CAD build for the part. Positions are in the model's coordinates, mm. A direction names the side the tool comes from. Coordinates: 2 decimals unless noted, no trailing zeros. Write each loop counter-clockwise with the first axis right and the second up, starting at its lowest first coordinate (ties: lowest second). Pieces come first, ordered by that corner, then holes. Notation, with made-up numbers: M 46.5,-9 L 90.5,-9 A14 ccw 90.5,-5 Z; hole C -20,-36 d1. An arc over 180 degrees is marked long. Answer as CSV lines item,"result". Start each with the question number.
```python
from build123d import *

# Parameters (mm, degrees)
BOSS_EXTRU_1_DEPTH      = 132
ESQUISSE3_W             = 4.94012132
ESQUISSE3_H             = 40
ENL_V_MAT_EXTRU_2_DEPTH = 9
ESQUISSE4_R             = 1.3
ENL_V_MAT_EXTRU_3_DEPTH = 18
ESQUISSE5_W             = 6
ESQUISSE5_H             = 24
ENL_V_MAT_EXTRU_4_DEPTH = 8
BOSS_EXTRU_2_REACH      = 38.8
ESQUISSE7_W             = 2
ESQUISSE7_H             = 18
ENL_V_MAT_EXTRU_5_DEPTH = 15
ENL_V_MAT_EXTRU_6_DEPTH = 15
ESQUISSE10_W            = 5.625
ESQUISSE10_H            = 32
BOSS_EXTRU_3_DEPTH      = 17
ESQUISSE12_W            = 12
ESQUISSE12_H            = 8
BOSS_EXTRU_4_DEPTH      = 13
ESQUISSE14_W            = 11.349962924
ESQUISSE14_H            = 7.588006138
BOSS_EXTRU_5_DEPTH      = 6
ESQUISSE16_W            = 13.258712606
ESQUISSE16_H            = 4.272246905
ENL_V_MAT_EXTRU_7_DEPTH = 11
ESQUISSE17_W            = 15.613345165
ESQUISSE17_H            = 5.100882875
BOSS_EXTRU_6_DEPTH      = 11
BOSS_EXTRU_6_DEPTH_BACK = 11
ESQUISSE11_R            = 1.85
ESQUISSE11_R_2          = 1.3
ESQUISSE11_R_3          = 2.916438904
ENL_V_MAT_EXTRU_8_DEPTH = 8
CONG_1_R                = 5
ESQUISSE18_W            = 9.677736186
ESQUISSE18_H            = 8.253244783
ENL_V_MAT_EXTRU_9_DEPTH = 10
CONG_2_R                = 5


with BuildPart() as part:
    # Esquisse1 → Boss.-Extru.1 (new body)
    with BuildSketch(Plane.XY):
        with BuildLine():
            Line((-12.4, 0), (-18.4, 0))
            Line((-18.4, 0), (-18.4, 18))
            Line((-18.4, 18), (18.4, 18))
            Line((18.4, 18), (18.4, 0))
            Line((18.4, 0), (12.4, 0))
            ThreePointArc((12.4, 0), (0, 12.4), (-12.4, 0))
        make_face()
    extrude(amount=BOSS_EXTRU_1_DEPTH)

    # Esquisse3 → Enlèv. mat.-Extru.2 (cut)
    with BuildSketch(Plane.XZ.offset(-18)):
        with Locations((0, 66)):
            Rectangle(ESQUISSE3_W, ESQUISSE3_H)
    extrude(amount=ENL_V_MAT_EXTRU_2_DEPTH, mode=Mode.SUBTRACT)

    # Esquisse4 → Enlèv. mat.-Extru.3 (cut)
    with BuildSketch(Plane(origin=(0, 18, 0), x_dir=(1, 0, 0), z_dir=(0, 1, 0))):
        with Locations((15.4, -6)):
            Circle(ESQUISSE4_R)
        with Locations((15.4, -18)):
            Circle(ESQUISSE4_R)
        with Locations((-15.4, -6)):
            Circle(ESQUISSE4_R)
        with Locations((-15.4, -18)):
            Circle(ESQUISSE4_R)
        with Locations((15.4, -30)):
            Circle(ESQUISSE4_R)
        with Locations((-15.4, -30)):
            Circle(ESQUISSE4_R)
        with Locations((15.4, -42)):
            Circle(ESQUISSE4_R)
        with Locations((-15.4, -42)):
            Circle(ESQUISSE4_R)
        with Locations((15.4, -54)):
            Circle(ESQUISSE4_R)
        with Locations((-15.4, -54)):
            Circle(ESQUISSE4_R)
        with Locations((-15.4, -126)):
            Circle(ESQUISSE4_R)
        with Locations((-15.4, -114)):
            Circle(ESQUISSE4_R)
        with Locations((-15.4, -102)):
            Circle(ESQUISSE4_R)
        with Locations((-15.4, -90)):
            Circle(ESQUISSE4_R)
        with Locations((-15.4, -78)):
            Circle(ESQUISSE4_R)
        with Locations((15.4, -78)):
            Circle(ESQUISSE4_R)
        with Locations((15.4, -90)):
            Circle(ESQUISSE4_R)
        with Locations((15.4, -102)):
            Circle(ESQUISSE4_R)
        with Locations((15.4, -114)):
            Circle(ESQUISSE4_R)
        with Locations((15.4, -126)):
            Circle(ESQUISSE4_R)
    extrude(amount=-ENL_V_MAT_EXTRU_3_DEPTH, mode=Mode.SUBTRACT)

    # Esquisse5 → Enlèv. mat.-Extru.4 (cut)
    with BuildSketch(Plane(origin=(0, 18, 0), x_dir=(1, 0, 0), z_dir=(0, 1, 0))):
        with Locations((15.4, -12)):
            Rectangle(ESQUISSE5_W, ESQUISSE5_H)
        with Locations((-15.4, -120)):
            Rectangle(ESQUISSE5_W, ESQUISSE5_H)
        with Locations((-15.4, -12)):
            Rectangle(ESQUISSE5_W, ESQUISSE5_H)
        with Locations((15.4, -120)):
            Rectangle(ESQUISSE5_W, ESQUISSE5_H)
    extrude(amount=-ENL_V_MAT_EXTRU_4_DEPTH, mode=Mode.SUBTRACT)

    # Esquisse7 → Boss.-Extru.2 (add, up to next)
    with BuildSketch(Plane.ZY.offset(18.4), mode=Mode.PRIVATE) as boss_extru_2_sk1:
        with Locations((66, 9)):
            Rectangle(ESQUISSE7_W, ESQUISSE7_H)
    boss_extru_2_tool1 = extrude(boss_extru_2_sk1.sketch, amount=-BOSS_EXTRU_2_REACH, mode=Mode.PRIVATE) - part.part
    add(boss_extru_2_tool1.solids().sort_by_distance((-18.4, 9, 66))[0])

    # Esquisse8 → Enlèv. mat.-Extru.5 (cut)
    with BuildSketch(Plane(origin=(0, 0, 65), x_dir=(-1, 0, 0), z_dir=(0, 0, -1))):
        with BuildLine():
            Line((12.775, 0), (-12.775, 0))
            ThreePointArc((-12.775, 0), (0, 12.775), (12.775, 0))
        make_face()
    extrude(amount=ENL_V_MAT_EXTRU_5_DEPTH, mode=Mode.SUBTRACT)

    # Esquisse9 → Enlèv. mat.-Extru.6 (cut)
    with BuildSketch(Plane.XY.offset(67)):
        with BuildLine():
            Line((12.775, 0), (-12.775, 0))
            ThreePointArc((-12.775, 0), (0, 12.775), (12.775, 0))
        make_face()
    extrude(amount=ENL_V_MAT_EXTRU_6_DEPTH, mode=Mode.SUBTRACT)

    # Esquisse10 → Boss.-Extru.3 (add)
    with BuildSketch(Plane.XZ):
        with Locations((15.5875, 66)):
            Rectangle(ESQUISSE10_W, ESQUISSE10_H)
        with Locations((-15.5875, 66)):
            Rectangle(ESQUISSE10_W, ESQUISSE10_H)
    extrude(amount=BOSS_EXTRU_3_DEPTH)

    # Esquisse12 → Boss.-Extru.4 (add)
    with BuildSketch(Plane(origin=(18.4, 0, 0), x_dir=(0, 0, -1), z_dir=(1, 0, 0))):
        with Locations((-102, 14)):
            Rectangle(ESQUISSE12_W, ESQUISSE12_H)
    extrude(amount=BOSS_EXTRU_4_DEPTH)

    # Esquisse14 → Boss.-Extru.5 (add)
    with BuildSketch(Plane(origin=(18.4, 0, 0), x_dir=(0, 0, -1), z_dir=(1, 0, 0))):
        with Locations((-50.7944077, 14.205996931)):
            Rectangle(ESQUISSE14_W, ESQUISSE14_H)
    extrude(amount=BOSS_EXTRU_5_DEPTH)

    # Esquisse16 → Enlèv. mat.-Extru.7 (cut)
    with BuildSketch(Plane(origin=(24.4, 0, 0), x_dir=(0, 0, -1), z_dir=(1, 0, 0))):
        with Locations((-50.566594151, 10.91391733)):
            Rectangle(ESQUISSE16_W, ESQUISSE16_H)
    extrude(amount=-ENL_V_MAT_EXTRU_7_DEPTH, mode=Mode.SUBTRACT)

    # Esquisse17 → Boss.-Extru.6 (add, two sides)
    with BuildSketch(Plane(origin=(18.4, 0, 0), x_dir=(0, 0, -1), z_dir=(1, 0, 0))) as boss_extru_6_sk:
        with Locations((-21.308135783, 15.449558563)):
            Rectangle(ESQUISSE17_W, ESQUISSE17_H)
    extrude(amount=BOSS_EXTRU_6_DEPTH)
    extrude(boss_extru_6_sk.sketch, amount=-BOSS_EXTRU_6_DEPTH_BACK)

    # Esquisse11 → Enlèv. mat.-Extru.8 (cut)
    with BuildSketch(Plane(origin=(0, 18, 0), x_dir=(1, 0, 0), z_dir=(0, 1, 0))):
        with Locations((24.22, -102)):
            Circle(ESQUISSE11_R)
        with Locations((19.13, -51)):
            Circle(ESQUISSE11_R)
        with Locations((24.22, -20.6)):
            Circle(ESQUISSE11_R)
        with Locations((-8.37, -51)):
            Circle(ESQUISSE11_R)
        with Locations((15.4, -6)):
            Circle(ESQUISSE11_R_2)
        with Locations((15.4, -18)):
            Circle(ESQUISSE11_R_3)
    extrude(amount=-ENL_V_MAT_EXTRU_8_DEPTH, mode=Mode.SUBTRACT)

    # Congé1
    cong_1_edges = [part.edges().sort_by_distance(p)[0] for p in [
        (29.4, 15.449558563, 13.5014632),
        (24.4, 15.525020391, 45.119426238),
        (24.4, 15.525020391, 56.469389162),
        (31.4, 14, 96),
        (31.4, 14, 108),
        (29.4, 15.449558563, 29.114808365),
    ]]
    fillet(cong_1_edges, radius=CONG_1_R)

    # Esquisse18 → Enlèv. mat.-Extru.9 (cut)
    with BuildSketch(Plane(origin=(-2.47006066, 0, 0), x_dir=(0, 0, -1), z_dir=(1, 0, 0))):
        with Locations((-50.900131157, 9.01339788)):
            Rectangle(ESQUISSE18_W, ESQUISSE18_H)
    extrude(amount=-ENL_V_MAT_EXTRU_9_DEPTH, mode=Mode.SUBTRACT)

    # Congé2
    cong_2_edges = [part.edges().sort_by_distance(p)[0] for p in [
        (0, 18, 0),
        (0, 18, 132),
    ]]
    fillet(cong_2_edges, radius=CONG_2_R)


solid = part.part
```
1) Pin check, flat tips, straight feed: P1, Ø6.5, axis at y = 14.5, z = 78, coming from the +X side; P2, Ø2, axis at x = -13, z = 42, coming from the -Y side; P3, Ø5, axis at x = -4, z = 16, coming from the -Y side. Stop position of each tip, or through.
2) Probe L1, parallel to X at y = 3.5, z = 41.5; L2, parallel to Z at x = 19.13, y = 15.75; L3, parallel to X at y = 4, z = 54. List the from-to ranges inside material, lowest first. Write a range as [from, to].
3) Two-plate mould, pull along Y, no slides. Class faces 1 (the flat face through (-15, 0, 107)), 2 (the flat face through (18, 13.05, 49)), 3 (the cylindrical face through (18.7, 15.6, 52.8)): pulls with the +Y half, pulls with the -Y half, needs draft (parallel to the pull), parting line crosses it, or undercut.
4) Tool access for faces 4 (the cylindrical face through (16.97, 15.49, 15.54)), 5 (the flat face through (19, 14, 108)), 6 (the flat face through (-12.775, -8, 66)): list every direction of +Z, -Z, +X, -X, +Y, -Y with a clear straight run to the whole face (end or side of a thin tool).
5) Band-saw the part on B-B, the plane z = 114. List the corners of the cut face in (x, y).
6) Band-saw the part on C-C, the plane x = 0. List the corners of the cut face in (y, z), plus the area to 3 significant figures.
7) Band-saw the part on A-A, the plane y = -5. List the corners of the cut face in (x, z) (3 decimals), plus the area to 3 significant figures.
8) Band-saw the part on D-D, the plane z = 78. List the corners of the cut face in (x, y) (3 decimals).
Result sheet:
1,P1,"stops at x = 18.4"
1,P2,"stops at y = 0"
1,P3,"stops at y = 10.56"
2,L1,"x = [-18.4, -16.6], [-14.2, -11.9], [11.9, 14.2], [16.6, 18.4]"
2,L2,"z = [13.5, 29.11], [45.12, 49.15], [52.85, 56.47], [96, 108]"
2,L3,"x = [-18.4, -16.7], [-14.1, -12.13], [12.13, 14.1], [16.7, 18.4]"
3,face 1,"pulls with the -Y half"
3,face 2,"undercut"
3,face 3,"needs draft"
4,face 4,"+Y"
4,face 5,"+Z, +X, +Y"
4,face 6,"+Z, -Z, -Y"
5,outline,"M -18.4,0 L -16.7,0 L -16.7,10 L -18.4,10 Z; M -14.1,0 L -12.4,0 A12.4 cw 12.4,0 L 14.1,0 L 14.1,10 L 12.4,10 L 12.4,18 L -12.4,18 L -12.4,10 L -14.1,10 Z; M 16.7,0 L 18.4,0 L 18.4,10 L 16.7,10 Z"
6,outline,"M 0,65 L 18,65 L 18,67 L 0,67 Z; M 12.4,0 L 13,0 A5 ccw 18,5 L 18,46 L 12.4,46 Z; M 12.4,86 L 18,86 L 18,127 A5 ccw 13,132 L 12.4,132 Z"
6,area,"540 mm²"
7,outline,"M -18.4,50 L -12.775,50 L -12.775,82 L -18.4,82 Z; M 12.775,50 L 18.4,50 L 18.4,82 L 12.775,82 Z"
7,area,"360 mm²"
8,outline,"M -18.4,-17 L -12.775,-17 L -12.775,0 A12.775 cw -2.47,12.534 L -2.47,18 L -14.1,18 L -14.1,0 L -16.7,0 L -16.7,18 L -18.4,18 Z; M 2.47,12.534 A12.775 cw 12.775,0 L 12.775,-17 L 18.4,-17 L 18.4,18 L 16.7,18 L 16.7,0 L 14.1,0 L 14.1,18 L 2.47,18 Z"
